```python
from build123d import *

# Parameters (mm, degrees)
CROQUIS1_W              = 900
CROQUIS1_H              = 1190.8
CROQUIS1_W_2            = 610
CROQUIS1_H_2            = 1120
SALIENTE_EXTRUIR1_DEPTH = 1.9
CROQUIS2_W              = 900
CROQUIS2_H              = 270
SALIENTE_EXTRUIR2_DEPTH = 1.9
CROQUIS4_W              = 800
CROQUIS4_H              = 220
CORTAR_EXTRUIR1_DEPTH   = 1.9
CROQUIS6_W              = 610
CROQUIS6_H              = 15
CORTAR_EXTRUIR2_DEPTH   = 10
CROQUIS7_W              = 800
CROQUIS7_H              = 14.9
SALIENTE_EXTRUIR3_DEPTH = 1.9
SALIENTE_EXTRUIR4_DEPTH = 1.9


with BuildPart() as part:
    # Croquis1 → Saliente-Extruir1 (new body)
    with BuildSketch(Plane.XY):
        with Locations((-450, 595.4)):
            Rectangle(CROQUIS1_W, CROQUIS1_H)
        with Locations((-450, 610.8)):
            Rectangle(CROQUIS1_W_2, CROQUIS1_H_2, mode=Mode.SUBTRACT)
    extrude(amount=SALIENTE_EXTRUIR1_DEPTH)

    # Croquis2 → Saliente-Extruir2 (add)
    with BuildSketch(Plane.XY.offset(1.9)):
        with Locations((-450, 1325.8)):
            Rectangle(CROQUIS2_W, CROQUIS2_H)
    extrude(amount=-SALIENTE_EXTRUIR2_DEPTH)

    # Croquis4 → Cortar-Extruir1 (cut)
    with BuildSketch(Plane.XY.offset(1.9)):
        with Locations((-450, 1315.8)):
            Rectangle(CROQUIS4_W, CROQUIS4_H)
    extrude(amount=-CORTAR_EXTRUIR1_DEPTH, mode=Mode.SUBTRACT)

    # Croquis6 → Cortar-Extruir2 (cut)
    with BuildSketch(Plane.XY.offset(1.9)):
        with Locations((-450, 1178.3)):
            Rectangle(CROQUIS6_W, CROQUIS6_H)
    extrude(amount=-CORTAR_EXTRUIR2_DEPTH, mode=Mode.SUBTRACT)

    # Croquis7 → Saliente-Extruir3 (add)
    with BuildSketch(Plane.XY.offset(1.9)):
        with Locations((-450, 1418.35)):
            Rectangle(CROQUIS7_W, CROQUIS7_H)
    extrude(amount=-SALIENTE_EXTRUIR3_DEPTH)

    # Croquis8 → Saliente-Extruir4 (add)
    with BuildSketch(Plane(origin=(0, 0, 0), x_dir=(-1, 0, 0), z_dir=(0, 0, -1))):
        Polygon((0, 1998), (0, 1460.8), (50.800000001, 1460.8), (50.8, 1947.2), (849.2, 1947.2), (849.200000001, 1460.8), (900, 1460.8), (900, 1998), align=None)
    extrude(amount=-SALIENTE_EXTRUIR4_DEPTH)


solid = part.part
```
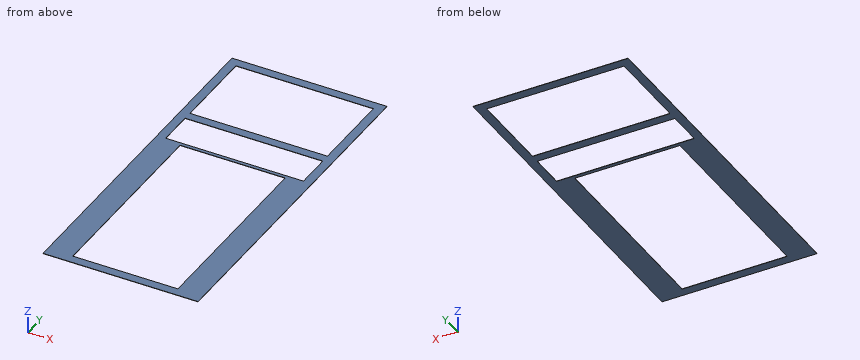
The model under review builds one solid part; all positions refer to its coordinate system, in mm. Round coordinates to 2 decimals unless told otherwise and drop trailing zeros. Order: outer loops, then holes, each group sorted by start corner. A loop starts at its lowest first (then second) coordinate and runs counter-clockwise, first axis right, second up. Notation, with made-up numbers: M -18,-11.5 L -8,-11.5 A3 cw -8,-7.5 Z; hole C -24,-31 d4. An arc over 180 degrees is marked long. Use a Markdown table: item, result.
1) Consider section B-B (y = 1288). Write out the cut boundary in (x, z).
Report:
| item | result |
|---|---|
| outline | M -900,0 L -850,0 L -850,1.9 L -900,1.9 Z; M -50,0 L 0,0 L 0,1.9 L -50,1.9 Z |
2) Consider section A-A (x = -456). Write out the cut boundary in (y, z).
Report:
| item | result |
|---|---|
| outline | M 0,0 L 50.8,0 L 50.8,1.9 L 0,1.9 Z; M 1185.8,0 L 1205.8,0 L 1205.8,1.9 L 1185.8,1.9 Z; M 1410.9,0 L 1460.8,0 L 1460.8,1.9 L 1410.9,1.9 Z; M 1947.2,0 L 1998,0 L 1998,1.9 L 1947.2,1.9 Z |
3) Wall thickness on line 1 along Y through (x, z) = (-812.5, 0.6); line 2 along Y through (x, z) = (-669.5, 1.05); line 3 along X through (y, z) = (337, 0.65): over which ranges is each line inside the solid? List them lowest first. Write a range as [from, to].
Report:
| item | result |
|---|---|
| line 1 | [0, 1205.8], [1410.9, 1460.8], [1947.2, 1998] |
| line 2 | [0, 50.8], [1185.8, 1205.8], [1410.9, 1460.8], [1947.2, 1998] |
| line 3 | [-900, -755], [-145, 0] |
4) Consider section D-D (y = 282). Write out the cut boundary in (x, z).
Report:
| item | result |
|---|---|
| outline | M -900,0 L -755,0 L -755,1.9 L -900,1.9 Z; M -145,0 L 0,0 L 0,1.9 L -145,1.9 Z |
5) Consider section C-C (z = 0.55). Write out the cut boundary in (x, y), then the cut area to 3 significant figures.
Report:
| item | result |
|---|---|
| outline | M -900,0 L 0,0 L 0,1998 L -900,1998 Z; hole M -850,1205.8 L -50,1205.8 L -50,1410.9 L -850,1410.9 Z; hole M -849.2,1460.8 L -50.8,1460.8 L -50.8,1947.2 L -849.2,1947.2 Z; hole M -755,50.8 L -145,50.8 L -145,1185.8 L -755,1185.8 Z |
| area | 553,000 mm^2 |
